The listing builds one solid part. Answer for the finished solid, in the listing's coordinates (mm). Face numbers are marked on the shaded views. Round coordinates to 2 decimals unless told otherwise and drop trailing zeros. Write each loop counter-clockwise with the first axis right and the second up, starting at its lowest first coordinate (ties: lowest second). Pieces come first, ordered by that corner, then holes.
Item 1: For a pull along Y with two mould halves and no side action, classify the marked faces 1, 2 and 3 as +Y half, -Y half, draft (parallel to the pull), parting line (faces both ways), or undercut.
Item 2: Each of these flat-tipped pins is pushed along its axis until it touches: pin 1 (2 mm diameter, centred on x = -4, y = -4, fed in from -Z); pin 2 (8 mm diameter, centred on y = -14.5, z = 12.5, fed in from -X); pin 3 (2 mm diameter, centred on y = -2, z = 48, fed in from +X). Where does it stop, or does it pass through?
Item 3: Find section A-A on y = 0. Give the vertices of the cut face in (x, z), then the cut area to 3 significant figures.
Item 4: Find the intervals of material crossed by probe 1 along Y at (x, z) = (0, 45); probe 2 along Z at (x, y) = (-4, -9); probe 3 along Y at (x, z) = (-7.5, 47), in increasing order.
Item 5: Find section C-C on z = 53. Give the vertices of the cut face in (x, y).
```python
from build123d import *

# Parameters (mm, degrees)
F0_R     = 19
F1_DEPTH = 135
F2_R     = 4
F3_R     = 19
F4_DEPTH = 7.5
F5_R     = 15
F6_DEPTH = 135.7
F7_R     = 2


with BuildPart() as f1:
    # F0 (on Top) → F1 (new body)
    with BuildSketch(Plane.XY):
        Circle(F0_R)
    extrude(amount=F1_DEPTH)

    # F2
    f2_edges = [f1.edges().sort_by_distance(p)[0] for p in [
        (-19, 0, 135),
    ]]
    fillet(f2_edges, radius=F2_R)

    # F3 (on Top) → F4 (join)
    with BuildSketch(Plane.XY):
        Circle(F3_R)
    extrude(amount=-F4_DEPTH)

    # F5 (on face) → F6 (cut)
    with BuildSketch(Plane(origin=(0, 0, -7.5), x_dir=(1, 0, 0), z_dir=(0, 0, -1))):
        Circle(F5_R)
    extrude(amount=-F6_DEPTH, mode=Mode.SUBTRACT)

    # F7
    f7_edges = [f1.edges().sort_by_distance(p)[0] for p in [
        (-19, 0, -7.5),
    ]]
    fillet(f7_edges, radius=F7_R)


solid = f1.part
```
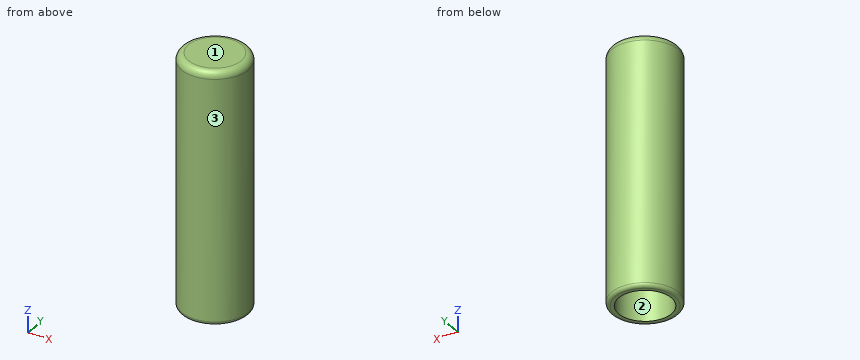
Check values:
1. face 1: draft
1. face 2: undercut
1. face 3: parting line
2. pin 1: stops at z = 128.2
2. pin 2: stops at x = -15.84
2. pin 3: stops at x = 18.97
3. outline: (-19, -5.5) arc R2 ccw to (-17, -7.5) - (-15, -7.5) - (-15, 128.2) - (15, 128.2) - (15, -7.5) - (17, -7.5) arc R2 ccw to (19, -5.5) - (19, 131) arc R4 ccw to (15, 135) - (-15, 135) arc R4 ccw to (-19, 131) - close
3. area: 1,340 mm2
4. probe 1: y = -19 to -15, 15 to 19
4. probe 2: z = 128.2 to 135
4. probe 3: y = -17.46 to -12.99, 12.99 to 17.46
5. outline: circle Ø38 at (0, 0); hole circle Ø30 at (0, 0)
